from build123d import *

# Parameters (mm, degrees)
F3_DEPTH = 20.32
F4_R     = 26.5969847408
F5_DEPTH = 254.001
F6_SCALE = 0.0393700787


with BuildPart() as f1:
    # F0 (on Front) → F1 (revolve)
    with BuildSketch(Plane.XZ):
        Polygon((-127, 0), (0, 0), (38.1, 0), (38.1, 50.8), (38.1, 76.2), (38.1, 101.6), (127, 101.6), (127, 127), (25.4, 127), (25.4, 101.6), (0, 101.6), (-25.4, 101.6), (-25.4, 127), (-127, 127), (-127, 101.6), (-38.1, 101.6), (-38.1, 76.2), (-38.1, 50.8), (-127, 50.8), (-127, 25.4), align=None)
    revolve(axis=Axis((-63.5, 0, 0), (-1, 0, 0)))

    # F2 (on face) → F3 (join)
    with BuildSketch(Plane.YZ.offset(38.1)):
        with BuildLine():
            ThreePointArc((50.4015624854, -6.3499999233), (50.7002927716, -3.1812439186), (50.8, 0))
            ThreePointArc((50.8, 0), (50.7002927716, 3.1812439186), (50.4015624854, 6.3499999233))
            ThreePointArc((50.4015624854, 6.3499999233), (35.9210244843, 35.9210244843), (6.3499999233, 50.4015624854))
            ThreePointArc((6.3499999233, 50.4015624854), (0, 50.8), (-6.3499999233, 50.4015624854))
            ThreePointArc((-6.3499999233, 50.4015624854), (-35.9210244843, 35.9210244843), (-50.4015624854, 6.3499999233))
            ThreePointArc((-50.4015624854, 6.3499999233), (-50.8, 0), (-50.4015624854, -6.3499999233))
            ThreePointArc((-50.4015624854, -6.3499999233), (-35.9210244843, -35.9210244843), (-6.3499999233, -50.4015624854))
            ThreePointArc((-6.3499999233, -50.4015624854), (0, -50.8), (6.3499999233, -50.4015624854))
            ThreePointArc((6.3499999233, -50.4015624854), (35.9210244843, -35.9210244843), (50.4015624854, -6.3499999233))
        make_face()
        with BuildLine():
            ThreePointArc((50.4015624854, 6.3499999233), (50.7002927716, 3.1812439186), (50.8, 0))
            ThreePointArc((50.8, 0), (50.7002927716, -3.1812439186), (50.4015624854, -6.3499999233))
            Line((50.4015624854, -6.3499999233), (101.4013683388, -6.3499999233))
            ThreePointArc((101.4013683388, -6.3499999233), (101.6, 0), (101.4013683388, 6.3499999233))
            Line((101.4013683388, 6.3499999233), (50.4015624854, 6.3499999233))
        make_face()
        with BuildLine():
            ThreePointArc((-6.3499999233, 50.4015624854), (0, 50.8), (6.3499999233, 50.4015624854))
            Line((6.3499999233, 50.4015624854), (6.3499999233, 101.4013683388))
            ThreePointArc((6.3499999233, 101.4013683388), (0, 101.6), (-6.3499999233, 101.4013683388))
            Line((-6.3499999233, 101.4013683388), (-6.3499999233, 50.4015624854))
        make_face()
        with BuildLine():
            Line((6.3499999233, -101.4013683388), (6.3499999233, -50.4015624854))
            ThreePointArc((6.3499999233, -50.4015624854), (0, -50.8), (-6.3499999233, -50.4015624854))
            Line((-6.3499999233, -50.4015624854), (-6.3499999233, -101.4013683388))
            ThreePointArc((-6.3499999233, -101.4013683388), (0, -101.6), (6.3499999233, -101.4013683388))
        make_face()
        with BuildLine():
            ThreePointArc((-50.4015624854, -6.3499999233), (-50.8, 0), (-50.4015624854, 6.3499999233))
            Line((-50.4015624854, 6.3499999233), (-101.4013683388, 6.3499999233))
            ThreePointArc((-101.4013683388, 6.3499999233), (-101.6, 0), (-101.4013683388, -6.3499999233))
            Line((-101.4013683388, -6.3499999233), (-50.4015624854, -6.3499999233))
        make_face()
    extrude(amount=F3_DEPTH)

    # F4 (on face) → F5 (cut, through all)
    with BuildSketch(Plane(origin=(-127, 0, 0), x_dir=(0, -1, 0), z_dir=(-1, 0, 0))):
        Circle(F4_R)
    extrude(amount=-F5_DEPTH, mode=Mode.SUBTRACT)


with BuildPart() as f1_1:
    # F6: moved
    add(f1.part.scale(F6_SCALE))


solid = f1_1.part
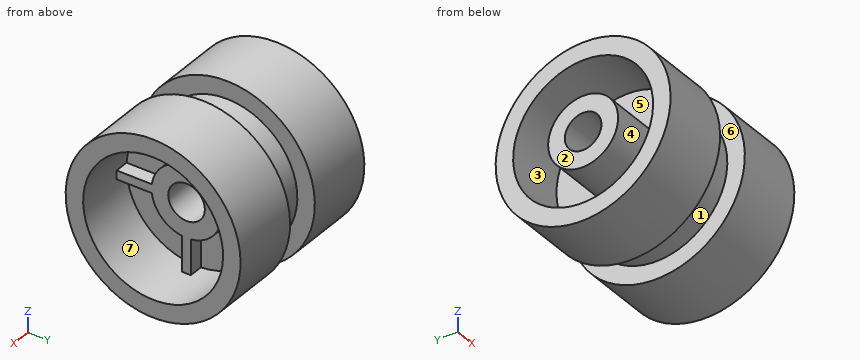
Could you check a few things on this model? Use its own coordinates, in mm. Face numbers are marked on the shaded views. A direction names the side the tool comes from. Give positions to 0.01 mm unless a question says otherwise; leave off trailing zeros. Order: outer loops, then holes, each group sorted by start corner. A loop starts at its lowest first (then second) coordinate and runs counter-clockwise, first axis right, second up. Notation, with made-up numbers: (85.25, 62.5) -> (134.25, 62.5) arc R20 cw to (134.25, 73.5) -> close; hole circle Ø9 at (-32.5, -40). An arc over 180 degrees is marked (long way). Answer in a Markdown table with one row per item. Add a question column.
Item 1: I'm going to push flat-ended pins straight in: P1, Ø3, axis at y = 0, z = -1.5, coming from the +X side; P2, Ø0.6, axis at x = 2, z = -3.5, coming from the -Y side; P3, Ø0.9, axis at x = 2, y = -3, coming from the +Z side. Where does each tip first touch, or does it pass through?
Item 2: We'd pull the mould along Z, two halves only. Please class the marked faces 1, 2, 3 and 4: pulls with the +Z half, pulls with the -Z half, needs draft (parallel to the pull), parting line crosses it, or undercut.
Item 3: Please list where these lines run through material, in increasing order: probe 1 along X at (y, z) = (4, -1.5); probe 2 along Y at (x, z) = (2.45, 0); probe 3 along Y at (x, z) = (2, 0.75).
Item 4: Imagine slicing it at A-A (y = 0). List the corners of the cut face in (x, z) for me.
Item 5: For the marked faces 5, 6 and 7, which set-ups out of +Z, -Z, +X, -X, +Y, -Y let a thin tool reach every point of the face, with its end or its side?
Item 6: Imagine slicing it at C-C (x = -4.5). List the corners of the cut face in (y, z) for me, and give its area (3 significant figures).
Item 7: Imagine slicing it at D-D (x = 3.5). List the corners of the cut face in (y, z) for me, and give its area (3 significant figures).
Result:
| question | item | result |
|---|---|---|
| 1 | P1 | x = 2.3 |
| 1 | P2 | y = -3.84 |
| 1 | P3 | z = 4.3 |
| 2 | face 1 | parting line crosses it |
| 2 | face 2 | needs draft |
| 2 | face 3 | undercut |
| 2 | face 4 | undercut |
| 3 | probe 1 | -5 to -1, 1 to 5 |
| 3 | probe 2 | -5 to -4, 4 to 5 |
| 3 | probe 3 | -4.94 to -3.93, -1.85 to -0.73, 0.73 to 1.85, 3.93 to 4.94 |
| 4 | outline | (-5, -5) -> (-1, -5) -> (-1, -4) -> (1, -4) -> (1, -5) -> (5, -5) -> (5, -4) -> (2.3, -4) -> (2.3, -1.05) -> (-5, -1.05) -> (-5, -2) -> (-1.5, -2) -> (-1.5, -4) -> (-5, -4) -> close; (-5, 1.05) -> (2.3, 1.05) -> (2.3, 4) -> (5, 4) -> (5, 5) -> (1, 5) -> (1, 4) -> (-1, 4) -> (-1, 5) -> (-5, 5) -> (-5, 4) -> (-1.5, 4) -> (-1.5, 2) -> (-5, 2) -> close |
| 5 | face 5 | -X |
| 5 | face 6 | none |
| 5 | face 7 | +X |
| 6 | outline | circle Ø10 at (0, 0); circle Ø4 at (0, 0); hole circle Ø8 at (0, 0); hole circle Ø2.09 at (0, 0) |
| 6 | area | 37.4 mm2 |
| 7 | outline | circle Ø10 at (0, 0); hole circle Ø8 at (0, 0) |
| 7 | area | 28.3 mm2 |
